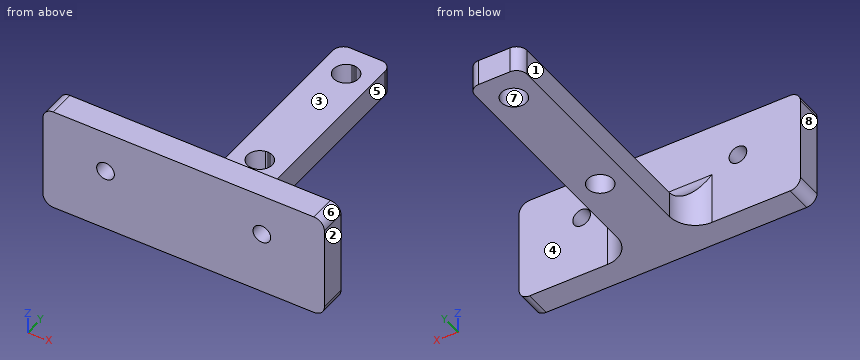
from build123d import *

# Parameters (mm, degrees)
SKETCH1_W               = 54
SKETCH1_H               = 20
BOSS_EXTRUDE1_DEPTH     = 5
BOSS_EXTRUDE2_OUTLINE_W = 10
BOSS_EXTRUDE2_OUTLINE_H = 5
BOSS_EXTRUDE2_DEPTH     = 50
M3_CLEARANCE_HOLE2_D    = 3.4
FILLET1_R               = 2
CUT_EXTRUDE6_DEPTH      = 13
CUT_EXTRUDE8_DEPTH      = 13
FILLET3_R               = 5


# Read off the part's stored shape, not the designer's step: Boss-Extrude2
with BuildPart() as part:
    # Sketch1 → Boss-Extrude1 (new body)
    with BuildSketch(Plane(origin=(0, 0, 0), x_dir=(1, 0, 0), z_dir=(0, 1, 0))):
        Rectangle(SKETCH1_W, SKETCH1_H)
    extrude(amount=BOSS_EXTRUDE1_DEPTH)

    # Boss-Extrude2 outline → Boss-Extrude2 (add)
    with BuildSketch(Plane(origin=(0, 5, 0), x_dir=(1, 0, 0), z_dir=(0, 1, 0))):
        with Locations((0, 7.5)):
            Rectangle(BOSS_EXTRUDE2_OUTLINE_W, BOSS_EXTRUDE2_OUTLINE_H)
    extrude(amount=BOSS_EXTRUDE2_DEPTH)

    # M3 Clearance Hole2 (through all)
    with Locations(Plane(origin=(0, 5, 0), x_dir=(1, 0, 0), z_dir=(0, 1, 0))):
        with Locations((15, -2), (-15, -2)):
            Hole(M3_CLEARANCE_HOLE2_D / 2)

    # Fillet1
    fillet1_edges = [part.edges().sort_by_distance(p)[0] for p in [
        (27, 2.5, 10),
        (-27, 2.5, 10),
        (5, 55, -7.5),
        (-5, 55, -7.5),
        (-27, 2.5, -10),
        (27, 2.5, -10),
    ]]
    fillet(fillet1_edges, radius=FILLET1_R)

    # Sketch16 → Cut-Extrude6 (cut)
    with BuildSketch(Plane.XY.offset(-5)):
        with BuildLine():
            Line((0, 51.537856262), (-0.416755626, 51.464371001))
            ThreePointArc((-0.416755626, 51.464371001), (0, 46.700832394), (0.416755626, 51.464371001))
            Line((0.416755626, 51.464371001), (0, 51.537856262))
        make_face()
    extrude(amount=-CUT_EXTRUDE6_DEPTH, mode=Mode.SUBTRACT)

    # Sketch17 → Cut-Extrude8 (cut)
    with BuildSketch(Plane.XY.offset(-5)):
        with BuildLine():
            Line((0, 25.437023869), (-0.416755626, 25.363538607))
            ThreePointArc((-0.416755626, 25.363538607), (0, 20.6), (0.416755626, 25.363538607))
            Line((0.416755626, 25.363538607), (0, 25.437023869))
        make_face()
    extrude(amount=-CUT_EXTRUDE8_DEPTH, mode=Mode.SUBTRACT)

    # Fillet3
    fillet3_edges = [part.edges().sort_by_distance(p)[0] for p in [
        (-5, 5, -7.5),
        (0, 5, -5),
        (5, 5, -7.5),
    ]]
    fillet(fillet3_edges, radius=FILLET3_R)


solid = part.part
Read the model definition and answer for the solid it produces. Units are mm, in the model's axes. Face numbers are marked on the shaded views. A direction names the side the tool comes from. Coordinates: 2 decimals unless noted, no trailing zeros. Loops run counter-clockwise (first coordinate to the right, second up) from the corner with the lowest first, then second, coordinate; pieces in that order, holes last. Notation, with made-up numbers: (55.5, 22) -> (64.5, 22) arc R19 cw to (64.5, 37) -> close; hole circle Ø5 at (65, 86). An arc over 180 degrees is marked (long way). Answer in a Markdown table with one row per item.
Item 1: A cutting plane is placed at C-C on x = 15. Determine the outline of the cut face in (y, z), plus the area to 3 significant figures.
Returned:
| item | result |
|---|---|
| outline | (0, -10) -> (5, -10) -> (5, 0.3) -> (0, 0.3) -> close; (0, 3.7) -> (5, 3.7) -> (5, 10) -> (0, 10) -> close |
| area | 83.0 mm^2 |
Item 2: A cutting plane is placed at B-B on z = 2. Determine the outline of the cut face in (x, y), plus the area to 3 significant figures.
Returned:
| item | result |
|---|---|
| outline | (-27, 0) -> (-16.7, 0) -> (-16.7, 5) -> (-27, 5) -> close; (-13.3, 0) -> (13.3, 0) -> (13.3, 5) -> (-13.3, 5) -> close; (16.7, 0) -> (27, 0) -> (27, 5) -> (16.7, 5) -> close |
| area | 236 mm^2 |
Item 3: A cutting plane is placed at D-D on z = -7. Determine the outline of the cut face in (x, y).
Returned:
| item | result |
|---|---|
| outline | (-27, 0) -> (27, 0) -> (27, 5) -> (10, 5) arc R5 cw to (5, 10) -> (5, 53) arc R2 ccw to (3, 55) -> (-3, 55) arc R2 ccw to (-5, 53) -> (-5, 10) arc R5 cw to (-10, 5) -> (-27, 5) -> close; hole (-0.42, 25.36) arc R2.4 ccw (long way) to (0.42, 25.36) -> (0, 25.44) -> close; hole (-0.42, 51.46) arc R2.4 ccw (long way) to (0.42, 51.46) -> (0, 51.54) -> close |
Item 4: For the marked faces 1, 2, 3, 4 and 5, determine the directions among +Z, -Z, +X, -X, +Y, -Y from which every point of the face is accessible in a straight line to the end or side of a thin tool.
Returned:
| item | result |
|---|---|
| face 1 | +Z, -Z, -X, +Y |
| face 2 | +Z, -Z, +X, +Y, -Y |
| face 3 | +Z, +X, -X, +Y |
| face 4 | +Z, +Y |
| face 5 | +Z, -Z, +X, +Y |
Item 5: Straight lines are drawn through the part: line 1 along Y through (x, z) = (0, -7.7); line 2 along Z through (x, y) = (15, 2.15); line 3 along X through (y, z) = (19, -6). For each, find the intervals that lie inside material, in ascending order. Write a range as [from, to].
Returned:
| item | result |
|---|---|
| line 1 | y = [0, 20.6], [25.44, 46.7], [51.54, 55] |
| line 2 | z = [-10, 0.3], [3.7, 10] |
| line 3 | x = [-5, 5] |
Item 6: For a pull along X with two mould halves and no side action, classify the marked faces 6, 7 and 8 as released by +X, released by -X, zero draft, split by the parting line, or undercut.
Returned:
| item | result |
|---|---|
| face 6 | released by +X |
| face 7 | undercut |
| face 8 | released by -X |
Item 7: A cutting plane is placed at A-A on y = 23. Determine the outline of the cut face in (x, z), plus the area to 3 significant figures.
Returned:
| item | result |
|---|---|
| outline | (-5, -10) -> (-2.4, -10) -> (-2.4, -5) -> (-5, -5) -> close; (2.4, -10) -> (5, -10) -> (5, -5) -> (2.4, -5) -> close |
| area | 26.0 mm^2 |
Item 8: Each of these flat-tipped pins is pushed along its axis until it touches: P1, Ø3, axis at y = 27.5, z = -3, coming from the -X side; P2, Ø4.5, axis at x = -15, z = 2, coming from the +Y side; P3, Ø6, axis at x = 0, y = 23, coming from the +Z side; P4, Ø5.5, axis at y = 21.5, z = -8.5, coming from the -X side. Where does it stop, or does it pass through?
Returned:
| item | result |
|---|---|
| P1 | passes through |
| P2 | stops at y = 5 |
| P3 | stops at z = -5 |
| P4 | stops at x = -5 |
